Model file for the job. Use its own axes, mm. Face numbers are marked on the shaded views. A direction names the side the tool comes from. Round coordinates to 2 decimals unless told otherwise and drop trailing zeros. Order: outer loops, then holes, each group sorted by start corner. A loop starts at its lowest first (then second) coordinate and runs counter-clockwise, first axis right, second up. Notation, with made-up numbers: (74.25, 8) -> (98.25, 8) arc R24 cw to (98.25, 41) -> close; hole circle Ø10 at (76, 0.5). An arc over 180 degrees is marked (long way). Answer as CSV lines item,"result".
```python
from build123d import *

# Parameters (mm, degrees)
SKETCH1_R           = 2
BOSS_EXTRUDE1_DEPTH = 2
CHAMFER1_SIZE       = 0.3
CUT_EXTRUDE1_DEPTH  = 1.5
CHAMFER2_SIZE       = 0.2
SKETCH3_R           = 1
BOSS_EXTRUDE2_DEPTH = 30
CHAMFER3_SIZE       = 0.2


with BuildPart() as part:
    # Sketch1 → Boss-Extrude1 (new body)
    with BuildSketch(Plane(origin=(0, 0, 0), x_dir=(1, 0, 0), z_dir=(0, 1, 0))):
        with Locations(Location((0, 0, 0), (0, 0, 270))):  # turned: the seam where the file's is
            Circle(SKETCH1_R)
    extrude(amount=BOSS_EXTRUDE1_DEPTH)

    # Chamfer1
    chamfer1_edges = [part.edges().sort_by_distance(p)[0] for p in [
        (0, 2, -2),
    ]]
    chamfer(chamfer1_edges, length=CHAMFER1_SIZE)

    # Sketch2 → Cut-Extrude1 (cut)
    with BuildSketch(Plane(origin=(0, 2, 0), x_dir=(1, 0, 0), z_dir=(0, 1, 0))):
        Polygon((1.154700538, 0), (0.577350269, 1), (-0.577350269, 1), (-1.154700538, 0), (-0.577350269, -1), (0.577350269, -1), align=None)
    extrude(amount=-CUT_EXTRUDE1_DEPTH, mode=Mode.SUBTRACT)

    # Chamfer2
    chamfer2_edges = [part.edges().sort_by_distance(p)[0] for p in [
        (0.866025404, 2, 0.5),
        (0.866025404, 2, -0.5),
        (0, 2, -1),
        (-0.866025404, 2, -0.5),
        (-0.866025404, 2, 0.5),
        (0, 2, 1),
    ]]
    chamfer(chamfer2_edges, length=CHAMFER2_SIZE)

    # Sketch3 → Boss-Extrude2 (add)
    with BuildSketch(Plane.XZ):
        with Locations(Location((0, 0, 0), (0, 0, 90))):  # turned: the seam where the file's is
            Circle(SKETCH3_R)
    extrude(amount=BOSS_EXTRUDE2_DEPTH)

    # Chamfer3
    chamfer3_edges = [part.edges().sort_by_distance(p)[0] for p in [
        (0, -30, -1),
    ]]
    chamfer(chamfer3_edges, length=CHAMFER3_SIZE)


solid = part.part
```
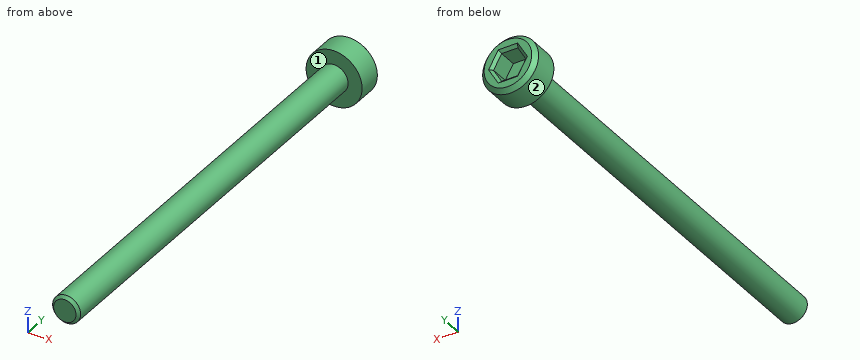
Q1. Tool access for the marked faces 1 and 2: list every direction of +Z, -Z, +X, -X, +Y, -Y with a clear straight run to the whole face (end or side of a thin tool).
Checks:
face 1,"-Y"
face 2,"+Y, -Y"
Q2. Wall check: L1, parallel to Y at x = 0.45, z = -0.6; L2, parallel to Y at x = -1.05, z = -0.6; L3, parallel to X at y = -11.5, z = 0. Give the ranges that are in metal, low to high. Write a range as [from, to].
Checks:
L1,"[-30, 0.5]"
L2,"[0, 2]"
L3,"[-1, 1]"
Q3. Saw through at A-A (x = 0). Write the cut outline in (y, z).
Checks:
outline,"(-30, -0.8) -> (-29.8, -1) -> (0, -1) -> (0, -2) -> (1.7, -2) -> (2, -1.7) -> (2, -1.2) -> (1.8, -1) -> (0.5, -1) -> (0.5, 1) -> (1.8, 1) -> (2, 1.2) -> (2, 1.7) -> (1.7, 2) -> (0, 2) -> (0, 1) -> (-29.8, 1) -> (-30, 0.8) -> close"
Q4. Saw through at B-B (y = -9.5). Write the cut outline in (x, z).
Checks:
outline,"circle Ø2 at (0, 0)"
Q5. Flat gauge pins, fed straight in: pin 1 (0.6 mm diameter, centred on x = -0.5, y = 1, fed in from -Z); pin 2 (2 mm diameter, centred on x = -1.5, z = 1.5, fed in from -Y); pin 3 (1.5 mm diameter, centred on y = -12, z = 0, fed in from +X). Where does each tip first touch, or does it go through?
Checks:
pin 1,"z = -1.99"
pin 2,"y = 0"
pin 3,"x = 1"
